```python
from build123d import *

# Parameters (mm, degrees)
SKETCH1_R           = 4.5
BOSS_EXTRUDE1_DEPTH = 53


with BuildPart() as part:
    # Sketch1 → Boss-Extrude1 (new body)
    with BuildSketch(Plane(origin=(0, 0, 0), x_dir=(1, 0, 0), z_dir=(0, 1, 0))):
        Polygon((-9.15, 14.65), (-10.65, 14.65), (-10.65, 10.65), (-14.65, 10.65), (-14.65, 9.15), (-12.65, 9.15), (-12.65, 7.65), (-11.15, 7.65), (-11.15, 0), (-11.15, -7.65), (-12.65, -7.65), (-12.65, -9.15), (-14.65, -9.15), (-14.65, -10.65), (-10.65, -10.65), (-10.65, -14.65), (-9.15, -14.65), (-9.15, -12.65), (-7.65, -12.65), (-7.65, -11.15), (0, -11.15), (7.65, -11.15), (7.65, -12.65), (9.15, -12.65), (9.15, -14.65), (10.65, -14.65), (10.65, -10.65), (14.65, -10.65), (14.65, -9.15), (12.65, -9.15), (12.65, -7.65), (11.15, -7.65), (11.15, 0), (11.15, 7.65), (12.65, 7.65), (12.65, 9.15), (14.65, 9.15), (14.65, 10.65), (10.65, 10.65), (10.65, 14.65), (9.15, 14.65), (9.15, 12.65), (7.65, 12.65), (7.65, 11.15), (0, 11.15), (-7.65, 11.15), (-7.65, 12.65), (-9.15, 12.65), align=None)
        with Locations(Location((-5.531430712, -5.531430712, 0), (0, 0, 270))):
            Circle(SKETCH1_R, mode=Mode.SUBTRACT)
        with Locations(Location((5.531430712, -5.531430712, 0), (0, 0, 270))):
            Circle(SKETCH1_R, mode=Mode.SUBTRACT)
        with Locations(Location((-5.531430712, 5.531430712, 0), (0, 0, 270))):
            Circle(SKETCH1_R, mode=Mode.SUBTRACT)
        with BuildLine():
            ThreePointArc((0, -1.7), (-1.202081528, -1.202081528), (-1.7, 0))
            ThreePointArc((-1.7, 0), (-1.202081528, 1.202081528), (0, 1.7))
            ThreePointArc((0, 1.7), (1.202081528, 1.202081528), (1.7, 0))
            ThreePointArc((1.7, 0), (1.202081528, -1.202081528), (0, -1.7))
        make_face(mode=Mode.SUBTRACT)
        with Locations(Location((5.531430712, 5.531430712, 0), (0, 0, 270))):
            Circle(SKETCH1_R, mode=Mode.SUBTRACT)
    extrude(amount=BOSS_EXTRUDE1_DEPTH)


solid = part.part
```
Could you check a few things on this model? Use its own coordinates, in mm. A direction names the side the tool comes from. Coordinates: 2 decimals unless noted, no trailing zeros. Write each loop counter-clockwise with the first axis right and the second up, starting at its lowest first coordinate (ties: lowest second). Pieces come first, ordered by that corner, then holes. Notation, with made-up numbers: (63, -2.75) -> (91, -2.75) arc R28 ccw to (91, 22.25) -> close; hole circle Ø9 at (7, 79.5). An arc over 180 degrees is marked (long way). Return JSON: item names as keys, results as strings.
(1) I need wall thicknesses on L1, parallel to X at y = 51.5, z = -7.5; L2, parallel to Z at x = -13, y = 37.5; L3, parallel to Z at x = 5, y = 50.5. Which ranges of each line are inside material? Lowest first, please.
Numbers:
{"L1": "x = -11.15 to -9.58, -1.48 to 1.48, 9.58 to 11.15", "L2": "z = -10.65 to -9.15, 9.15 to 10.65", "L3": "z = -11.15 to -10, -1.06 to 1.06, 10 to 11.15"}
(2) I'm going to push flat-ended pins straight in: pin 1 (1.2 mm diameter, centred on y = 35.5, z = -12.5, fed in from -X); pin 2 (3 mm diameter, centred on x = -6.5, y = 41.5, fed in from -Z); pin 3 (17 mm diameter, centred on y = 25, z = -0.5, fed in from -X); pin 4 (5.5 mm diameter, centred on x = 5.53, z = 5.53, fed in from +Y). Where does each tip first touch, or does it pass through?
Numbers:
{"pin 1": "stops at x = -10.65", "pin 2": "stops at z = -12.65", "pin 3": "stops at x = -12.65", "pin 4": "passes through"}
(3) Imagine slicing it at B-B, the plane x = -3. Please give me the cut outline in (y, z).
Numbers:
{"outline": "(0, -11.15) -> (53, -11.15) -> (53, -9.25) -> (0, -9.25) -> close; (0, -1.81) -> (53, -1.81) -> (53, 1.81) -> (0, 1.81) -> close; (0, 9.25) -> (53, 9.25) -> (53, 11.15) -> (0, 11.15) -> close"}
(4) Imagine slicing it at C-C, the plane y = 32. Count the separate pieces of the cut face and the enclosed holes in it, then the cut area to 3 significant figures.
Numbers:
{"separate pieces": "1", "enclosed holes": "5", "area": "293 mm2"}
(5) Imagine slicing it at A-A, the plane z = -6. Please give me the cut outline in (x, y), then the cut area to 3 significant figures.
Numbers:
{"outline": "(-11.15, 0) -> (-10.01, 0) -> (-10.01, 53) -> (-11.15, 53) -> close; (-1.06, 0) -> (1.06, 0) -> (1.06, 53) -> (-1.06, 53) -> close; (10.01, 0) -> (11.15, 0) -> (11.15, 53) -> (10.01, 53) -> close", "area": "233 mm2"}
(6) Which directions (+Z, -Z, +X, -X, +Y, -Y) give clear straight access to the entire face, cutting with the end or side of a thin tool? Please do faces 5 (the flat face through (12.65, 26, 8)), 6 (the flat face through (-7.65, 26, 12)), 7 (the flat face through (-12.65, 26, 8)), 8 (the flat face through (-9.15, 26, -14)), 9 (the flat face through (10, 26, 14.65)).
Numbers:
{"face 5": "+X, +Y, -Y", "face 6": "+Z, +Y, -Y", "face 7": "-X, +Y, -Y", "face 8": "-Z, +Y, -Y", "face 9": "+Z, +X, -X, +Y, -Y"}
(7) We'd pull the mould along X, two halves only. Please class faces 1 (the flat face through (-12, 26, -7.65)), 2 (the cylindrical face through (6.88, 26.13, -1.24)), 3 (the flat face through (7.65, 26, 12)), 4 (the flat face through (14.65, 26, -10)): +X half, -X half, draft (parallel to the pull), parting line (faces both ways), or undercut.
Numbers:
{"face 1": "draft", "face 2": "undercut", "face 3": "undercut", "face 4": "+X half"}
